Input: part model. Units: mm. Frame: model coordinates. A direction names the side the tool comes from. Coordinates: 2 decimals unless noted, no trailing zeros. Loops run counter-clockwise (first coordinate to the right, second up) from the corner with the lowest first, then second, coordinate; pieces in that order, holes last.
```python
from build123d import *

# Parameters (mm, degrees)
SKETCH1_W           = 35.5
SKETCH1_H           = 75.5
BOSS_EXTRUDE2_DEPTH = 23
CUT_EXTRUDE1_DEPTH  = 21
SKETCH2_W           = 4
SKETCH2_H           = 4
BOSS_EXTRUDE3_DEPTH = 9.3
CUT_EXTRUDE2_START  = -15.05
SKETCH3_W           = 3.25
SKETCH3_H           = 9
CUT_EXTRUDE2_DEPTH  = 4.25
SKETCH6_R           = 4.25
CUT_EXTRUDE4_DEPTH  = 1.75
FILLET1_R           = 1
FILLET2_R           = 1
SKETCH7_R           = 7.218245837
SKETCH7_R_2         = 5.218245837
BOSS_EXTRUDE4_DEPTH = 2
SKETCH9_R           = 7.218245837
BOSS_EXTRUDE5_DEPTH = 2
FILLET4_R           = 1
SKETCH10_R          = 4.340870449
CUT_EXTRUDE5_DEPTH  = 2
FILLET5_R           = 1
FILLET6_R           = 1
FILLET7_R           = 1
FILLET9_R           = 1
BOSS_EXTRUDE7_DEPTH = 10
FILLET10_R          = 1
SKETCH13_R          = 1.5
CUT_EXTRUDE6_DEPTH  = 21


with BuildPart() as part:
    # Sketch1 → Boss-Extrude2 (new body)
    with BuildSketch(Plane(origin=(0, 0, 0), x_dir=(1, 0, 0), z_dir=(0, 1, 0))):
        with Locations((17.75, 37.75)):
            Rectangle(SKETCH1_W, SKETCH1_H)
    extrude(amount=BOSS_EXTRUDE2_DEPTH)

    # 3DSketch1 → Cut-Extrude1 (cut)
    with BuildSketch(Plane(origin=(33.75, 23, -1.75), x_dir=(-0.40613846605344744, 0, -0.9138115486202573), z_dir=(0, 1, 0))):
        Polygon((0, 0), (65.794431501, -29.241969556), (78.790862414, 0), (12.996430914, 29.241969556), align=None)
    extrude(amount=-CUT_EXTRUDE1_DEPTH, mode=Mode.SUBTRACT)

    # Sketch2 → Boss-Extrude3 (add)
    with BuildSketch(Plane(origin=(0, 2, 0), x_dir=(1, 0, 0), z_dir=(0, 1, 0))):
        with Locations((3.75, 71.75)):
            Rectangle(SKETCH2_W, SKETCH2_H)
        with Locations((31.75, 71.75)):
            Rectangle(SKETCH2_W, SKETCH2_H)
        with Locations((31.75, 3.75)):
            Rectangle(SKETCH2_W, SKETCH2_H)
        with Locations((3.75, 3.75)):
            Rectangle(SKETCH2_W, SKETCH2_H)
    extrude(amount=BOSS_EXTRUDE3_DEPTH)

    # Sketch3 → Cut-Extrude2 (cut)
    with BuildSketch(Plane(origin=(0, 23, 0), x_dir=(1, 0, 0), z_dir=(0, 1, 0)).offset(CUT_EXTRUDE2_START)):
        with Locations((33.875, 30.8)):
            Rectangle(SKETCH3_W, SKETCH3_H)
    extrude(amount=-CUT_EXTRUDE2_DEPTH, mode=Mode.SUBTRACT)

    # Sketch6 → Cut-Extrude4 (cut)
    with BuildSketch(Plane.XY):
        with Locations((16.758366621, 11.3)):
            Circle(SKETCH6_R)
    extrude(amount=-CUT_EXTRUDE4_DEPTH, mode=Mode.SUBTRACT)

    # Fillet1
    fillet1_edges = [part.edges().sort_by_distance(p)[0] for p in [
        (12.508366621, 11.3, -1.75),
    ]]
    fillet(fillet1_edges, radius=FILLET1_R)

    # Fillet2
    # the kernel refuses this fillet: 1 mm, written as the material it takes off along each edge
    with BuildSketch(Plane(origin=(16.758366621, 11.3, 0), x_dir=(1, 0, 0), z_dir=(0, -1, 0))) as fillet2_piece_1:
        with BuildLine():
            CenterArc((5.218245837, -1), FILLET2_R, 90, 75.522487814)
            Line((5.218245837, 0), (5.218245837, 0.02))
            Line((5.218245837, 0.02), (4.25, 0.02))
            Line((4.25, 0.02), (4.23, 0))
            ThreePointArc((4.23, 0), (4.23, -0.375), (4.230635083, -0.745))
            Line((4.230635083, -0.745), (4.25, -0.75))
        make_face()
    revolve(axis=Axis((16.758366621, 11.3, 0), (0, 0, 1)), mode=Mode.SUBTRACT)

    # Sketch7 → Boss-Extrude4 (add)
    with BuildSketch(Plane.XY):
        with Locations(Location((16.758366621, 11.3, 0), (0, 0, 180))):
            Circle(SKETCH7_R)
        with Locations(Location((16.758366621, 11.3, 0), (0, 0, 180))):
            Circle(SKETCH7_R_2, mode=Mode.SUBTRACT)
    extrude(amount=BOSS_EXTRUDE4_DEPTH)

    # Sketch9 → Boss-Extrude5 (add)
    with BuildSketch(Plane.XY.offset(2)):
        with Locations(Location((16.758366621, 11.3, 0), (0, 0, 180))):
            Circle(SKETCH9_R)
    extrude(amount=BOSS_EXTRUDE5_DEPTH)

    # Fillet4
    fillet4_edges = [part.edges().sort_by_distance(p)[0] for p in [
        (23.976612458, 11.3, 4),
    ]]
    fillet(fillet4_edges, radius=FILLET4_R)

    # Sketch10 → Cut-Extrude5 (cut)
    with BuildSketch(Plane.XY.offset(4)):
        with Locations((16.758366621, 11.3)):
            Circle(SKETCH10_R)
    extrude(amount=-CUT_EXTRUDE5_DEPTH, mode=Mode.SUBTRACT)

    # Fillet5
    fillet5_edges = [part.edges().sort_by_distance(p)[0] for p in [
        (34.625, 3.7, -26.3),
    ]]
    fillet(fillet5_edges, radius=FILLET5_R)

    # Fillet6
    fillet6_edges = [part.edges().sort_by_distance(p)[0] for p in [
        (34.625, 3.7, -35.3),
    ]]
    fillet(fillet6_edges, radius=FILLET6_R)

    # Fillet7
    fillet7_edges = [part.edges().sort_by_distance(p)[0] for p in [
        (5.75, 6.65, -69.75),
        (29.75, 6.65, -69.75),
        (29.75, 6.65, -5.75),
        (5.75, 6.65, -5.75),
    ]]
    fillet(fillet7_edges, radius=FILLET7_R)

    # Fillet9
    fillet9_edges = [part.edges().sort_by_distance(p)[0] for p in [
        (34.625, 7.95, -26.3),
        (34.625, 7.95, -35.3),
    ]]
    fillet(fillet9_edges, radius=FILLET9_R)

    # Sketch12 → Boss-Extrude7 (add)
    with BuildSketch(Plane(origin=(35.5, 0, 0), x_dir=(0, 0, -1), z_dir=(1, 0, 0))):
        with BuildLine():
            Line((37.020541431, 11.65), (24.579458569, 11.65))
            ThreePointArc((24.579458569, 11.65), (23.872351788, 11.357106781), (23.579458569, 10.65))
            Line((23.579458569, 10.65), (23.579458569, 1))
            ThreePointArc((23.579458569, 1), (23.872351788, 0.292893219), (24.579458569, 0))
            Line((24.579458569, 0), (37.020541431, 0))
            ThreePointArc((37.020541431, 0), (37.727648212, 0.292893219), (38.020541431, 1))
            Line((38.020541431, 1), (38.020541431, 10.65))
            ThreePointArc((38.020541431, 10.65), (37.727648212, 11.357106781), (37.020541431, 11.65))
        make_face()
        with BuildLine():
            Line((35.3, 9.325), (26.3, 9.325))
            ThreePointArc((26.3, 9.325), (25.592893219, 9.032106781), (25.3, 8.325))
            Line((25.3, 8.325), (25.3, 3.325))
            ThreePointArc((25.3, 3.325), (25.592893219, 2.617893219), (26.3, 2.325))
            Line((26.3, 2.325), (35.3, 2.325))
            ThreePointArc((35.3, 2.325), (36.007106781, 2.617893219), (36.3, 3.325))
            Line((36.3, 3.325), (36.3, 8.325))
            ThreePointArc((36.3, 8.325), (36.007106781, 9.032106781), (35.3, 9.325))
        make_face(mode=Mode.SUBTRACT)
    extrude(amount=BOSS_EXTRUDE7_DEPTH)

    # Fillet10
    fillet10_edges = [part.edges().sort_by_distance(p)[0] for p in [
        (45.5, 0.292893219, -23.872351788),
        (45.5, 0, -30.8),
        (45.5, 0.292893219, -37.727648212),
        (45.5, 5.825, -38.020541431),
        (45.5, 11.357106781, -37.727648212),
        (45.5, 11.65, -30.8),
        (45.5, 11.357106781, -23.872351788),
        (45.5, 5.825, -23.579458569),
    ]]
    fillet(fillet10_edges, radius=FILLET10_R)

    # Sketch13 → Cut-Extrude6 (cut)
    with BuildSketch(Plane.XY.offset(-23.579458569)):
        with Locations((41.17, 5.31975288)):
            Circle(SKETCH13_R)
    extrude(amount=-CUT_EXTRUDE6_DEPTH, mode=Mode.SUBTRACT)


solid = part.part
```
Item 1: Section query B-B (z = -18). Output: boundary loops of the cut face in (x, y), then the cut area to 4 significant figures.
Result:
outline: (0, 0) - (35.5, 0) - (35.5, 23) - (33.75, 23) - (33.75, 2) - (1.75, 2) - (1.75, 23) - (0, 23) - close
area: 144.5 mm2
Item 2: Reachability of faces 4 (the face through (40, 2.325, -31)), 5 (the face through (39, 6, -23.579)), 6 (the face through (29.75, 7, -3)), 7 (the face through (20.899, 14.475, 0.986)) from +Z, -Z, +X, -X, +Y, -Y: full face, straight path, thin tool, end or side. Return the list, or none.
Result:
face 4: +X
face 5: +Z, +X, +Y, -Y
face 6: +Y
face 7: none
Item 3: Line query: L1, parallel to X at y = 22.25, z = -18.5; L2, parallel to Z at x = 33, y = 13.25; L3, parallel to Z at x = 40, y = 3.25. Output: solid intervals per line, ascending.
Result:
L1: x = 0 to 1.75, 33.75 to 35.5
L2: z = -75.5 to -73.75, -1.75 to 0
L3: z = -38.02 to -36.3, -25.3 to -23.58
Item 4: Contact query for flat-ended pins moving along their axis: P1, Ø1.2, axis at x = 31.5, z = -3.5, coming from the +Y side; P2, Ø4, axis at x = 40.5, y = 5.5, coming from the -Z side; P3, Ø1, axis at x = 35, y = 16.5, coming from the +Z side. Output: stop coordinate, or through.
Result:
P1: stops at y = 11.3
P2: stops at z = -38.02
P3: stops at z = 0
Item 5: Mould query, pull axis Z, two halves, no side actions, for faces 1 (the face through (18, 11, -75.5)), 2 (the face through (21, 13, 4)), 3 (the face through (18, 2, -37)). Classes: +Z half, -Z half, draft (parallel to the pull), parting line (faces both ways), or undercut.
Result:
face 1: -Z half
face 2: +Z half
face 3: undercut
Item 6: Section query A-A (x = 41.17). Output: boundary loops of the cut face in (y, z) (3 decimals), then the cut area to 3 significant figures.
Result:
outline: (0, -37.021) arc R1 ccw to (1, -38.021) - (3.82, -38.021) - (3.82, -36.3) - (3.325, -36.3) arc R1 cw to (2.325, -35.3) - (2.325, -26.3) arc R1 cw to (3.325, -25.3) - (3.82, -25.3) - (3.82, -23.579) - (1, -23.579) arc R1 ccw to (0, -24.579) - close; (6.82, -38.021) - (10.65, -38.021) arc R1 ccw to (11.65, -37.021) - (11.65, -24.579) arc R1 ccw to (10.65, -23.579) - (6.82, -23.579) - (6.82, -25.3) - (8.325, -25.3) arc R1 cw to (9.325, -26.3) - (9.325, -35.3) arc R1 cw to (8.325, -36.3) - (6.82, -36.3) - close
area: 80.9 mm2
